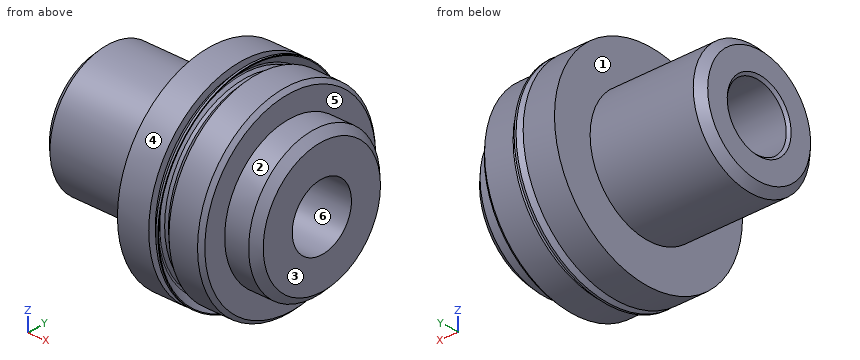
Autodesk Inventor part; units mm, degrees
ref_plane "hh_XY" through (0, 6.35, 0) normal (0, 0, 1) x (1, 0, 0)
ref_plane "hh_YZ" through (0, 6.35, 0) normal (1, 0, 0) x (0, 1, 0)
ref_plane "hh_ZX" through (0, 6.35, 0) normal (0, 1, 0) x (0, 0, 1)
sketch "Sketch_1" plane through (0, 0, 0) normal (0, 0, 1) x (1, 0, 0)
  line L0 (11.1252, 0) -> (0, 0)
  line L1 (0, 0) -> (0, 5.5944)
  line L2 (0, 5.5944) -> (0.7557, 6.35)
  line L3 (0.7557, 6.35) -> (11.1252, 6.35)
  line L4 (11.1252, 6.35) -> (11.1252, 0)
  line L5 (11.1252, 0) -> (0, 0)
revolve "Revolution1" add sketch "Sketch_1" angle 360 about axis through (11.1252, 0, 0) along (1, 0, 0)
thread "Thread1"
sketch "Sketch_3" plane through (0, 0, 0) normal (0, 0, 1) x (1, 0, 0)
  line L0 (19.05, 0) -> (11.1252, 0)
  line L1 (11.1252, 0) -> (11.1252, 10.2235)
  line L2 (11.1252, 10.2235) -> (14.2748, 10.2235)
  line L3 (14.2748, 10.2235) -> (14.2748, 8.9091)
  line L4 (14.2748, 8.9091) -> (15.0368, 8.9091)
  line L5 (15.0368, 8.9091) -> (15.7988, 9.671)
  line L6 (15.7988, 9.671) -> (18.669, 9.671)
  line L7 (18.669, 9.671) -> (19.05, 9.2901)
  line L8 (19.05, 9.2901) -> (19.05, 0)
  line L9 (19.05, 0) -> (11.1252, 0)
revolve "Revolution2" add sketch "Sketch_3" angle 360 about axis through (19.05, 0, 0) along (1, 0, 0)
sketch "Sketch_4" plane through (0, 0, 0) normal (0, 0, 1) x (1, 0, 0)
  line L0 (22.225, 0) -> (19.05, 0)
  line L1 (19.05, 0) -> (19.05, 7.1374)
  line L2 (19.05, 7.1374) -> (21.463, 7.1374)
  line L3 (21.463, 7.1374) -> (22.225, 6.3754)
  line L4 (22.225, 6.3754) -> (22.225, 0)
  line L5 (22.225, 0) -> (19.05, 0)
revolve "Revolution3" add sketch "Sketch_4" angle 360 about axis through (22.225, 0, 0) along (1, 0, 0)
sketch "Sketch4" plane through (0, 0, 0) normal (-1, 0, 0) x (0, 0, 1)
  point P0 (0, 0)
hole "Hole1" at (0, 0, 0) direction (1, 0, 0) diameter 6.4389 depth 22.225 countersink diameter 6.9469 countersink angle 90
sketch "Sketch_47" plane through (0, 0, 0) normal (0, 0, 1) x (1, 0, 0)
  line L0 (15.0368, 0) -> (14.2748, 0)
  line L1 (14.2748, 9.512) -> (14.2748, 8.655)
  line L2 (14.2748, 8.655) -> (15.0368, 8.655)
  line L3 (15.0368, 8.655) -> (15.0368, 8.9091)
  line L4 (15.0368, 8.9091) -> (14.6558, 8.9091)
  line L5 (14.6558, 8.9091) -> (14.3973, 9.1676)
  arc A0 (14.3973, 9.3472) -> (14.3973, 9.1676) centre (14.4871, 9.2574) ccw
  line L6 (14.3973, 9.3472) -> (15.1895, 10.1393)
  line L7 (15.1895, 10.1393) -> (15.1895, 10.2235)
  line L8 (15.1895, 10.2235) -> (14.9863, 10.2235)
  line L9 (14.9863, 10.2235) -> (14.2748, 9.512)
revolve "Revolution4" add sketch "Sketch_47" angle 360 about axis through (15.0368, 0, 0) along (1, 0, 0)
ref_plane "hh_XY" through (0, 6.35, 0) normal (0, 0, 1) x (1, 0, 0)
ref_plane "hh_YZ" through (0, 6.35, 0) normal (1, 0, 0) x (0, 1, 0)
ref_plane "hh_ZX" through (0, 6.35, 0) normal (0, 1, 0) x (0, 0, 1)
ref_plane "rod_guide_XY" through (0, 0, 0) normal (1, 0, 0) x (0, 0, -1)
ref_plane "rod_guide_YZ" through (0, 0, 0) normal (0, 0, -1) x (0, 1, 0)
ref_plane "rod_guide_ZX" through (0, 0, 0) normal (0, 1, 0) x (1, 0, 0)
ref_plane "t1_XY" through (11.1252, 0, 0) normal (1, 0, 0) x (0, 0, -1)
ref_plane "t1_YZ" through (11.1252, 0, 0) normal (0, 0, -1) x (0, 1, 0)
ref_plane "t1_ZX" through (11.1252, 0, 0) normal (0, 1, 0) x (1, 0, 0)
ref_plane "t111_XY" through (11.1252, 0, 0) normal (1, 0, 0) x (0, 0, -1)
ref_plane "t111_YZ" through (11.1252, 0, 0) normal (0, 0, -1) x (0, 1, 0)
ref_plane "t111_ZX" through (11.1252, 0, 0) normal (0, 1, 0) x (1, 0, 0)
ref_plane "to_foot_bracket_XY" through (11.1252, 0, 0) normal (1, 0, 0) x (0, 0, -1)
ref_plane "to_foot_bracket_YZ" through (11.1252, 0, 0) normal (0, 0, -1) x (0, 1, 0)
ref_plane "to_foot_bracket_ZX" through (11.1252, 0, 0) normal (0, 1, 0) x (1, 0, 0)
ref_plane "to_nut_XY" through (11.1252, 0, 0) normal (1, 0, 0) x (0, 0, -1)
ref_plane "to_nut_YZ" through (11.1252, 0, 0) normal (0, 0, -1) x (0, 1, 0)
ref_plane "to_nut_ZX" through (11.1252, 0, 0) normal (0, 1, 0) x (1, 0, 0)
ref_plane "to_rod_XY" through (0, 0, 0) normal (1, 0, 0) x (0, 0, -1)
ref_plane "to_rod_YZ" through (0, 0, 0) normal (0, 0, -1) x (0, 1, 0)
ref_plane "to_rod_ZX" through (0, 0, 0) normal (0, 1, 0) x (1, 0, 0)
ref_plane "to_screw_XY" through (6.35, 2.032, -6.0452) normal (0, 1, 0) x (1, 0, 0)
ref_plane "to_screw_YZ" through (6.35, 2.032, -6.0452) normal (1, 0, 0) x (0, 0, -1)
ref_plane "to_screw_ZX" through (6.35, 2.032, -6.0452) normal (0, 0, -1) x (0, 1, 0)
ref_plane "to_trunnion_brackets_XY" through (11.1252, 0, 0) normal (0, 1, 0) x (1, 0, 0)
ref_plane "to_trunnion_brackets_YZ" through (11.1252, 0, 0) normal (1, 0, 0) x (0, 0, -1)
ref_plane "to_trunnion_brackets_ZX" through (11.1252, 0, 0) normal (0, 0, -1) x (0, 1, 0)
ref_plane "to_trunnion_brackets1_XY" through (11.1252, 12.7, 0) normal (0, 1, 0) x (1, 0, 0)
ref_plane "to_trunnion_brackets1_YZ" through (11.1252, 12.7, 0) normal (1, 0, 0) x (0, 0, -1)
ref_plane "to_trunnion_brackets1_ZX" through (11.1252, 12.7, 0) normal (0, 0, -1) x (0, 1, 0)
ref_plane "to_trunnion_brackets2_XY" through (11.1252, -12.7, 0) normal (0, 1, 0) x (1, 0, 0)
ref_plane "to_trunnion_brackets2_YZ" through (11.1252, -12.7, 0) normal (1, 0, 0) x (0, 0, -1)
ref_plane "to_trunnion_brackets2_ZX" through (11.1252, -12.7, 0) normal (0, 0, -1) x (0, 1, 0)
ref_plane "to_tube_XY" through (15.0368, 0, 0) normal (1, 0, 0) x (0, 0, -1)
ref_plane "to_tube_YZ" through (15.0368, 0, 0) normal (0, 0, -1) x (0, 1, 0)
ref_plane "to_tube_ZX" through (15.0368, 0, 0) normal (0, 1, 0) x (1, 0, 0)
properties part number "04000-0_rod_guide"
Can you work these out from the model? Positions are in its coordinate system, mm. Face numbers are marked on the shaded views. A direction names the side the tool comes from. Give positions to 0.01 mm unless a question says otherwise; leave off trailing zeros. Order: outer loops, then holes, each group sorted by start corner. A loop starts at its lowest first (then second) coordinate and runs counter-clockwise, first axis right, second up. Notation, with made-up numbers: M -17.75,63.25 L 36.25,63.25 A27 ccw 36.25,89.25 Z; hole C -36.75,40 d11. An arc over 180 degrees is marked long. One line per item, written item: value.
Item 1: For the marked faces 1, 2 and 3, which set-ups out of +Z, -Z, +X, -X, +Y, -Y let a thin tool reach every point of the face, with its end or its side?
Verdict:
face 1: -X
face 2: +X
face 3: +Z, -Z, +X, +Y, -Y
Item 2: If we section it at A-A on x = 4.25: Write out the boundary of the cut face in (y, z).
Verdict:
outline: C 0,0 d12.7; hole C 0,0 d6.44
Item 3: If we mould it in two halves opening along Y, with no side actions, what happens to the marked faces 4, 5 and 6? For each: pulls with the +Y half, pulls with the -Y half, needs draft (parallel to the pull), parting line crosses it, or undercut.
Verdict:
face 4: parting line crosses it
face 5: needs draft
face 6: undercut
Item 4: Please list where these lines run through material, in increasing order: line 1 (Z direction, x = 11.75, y = 0); line 2 (Z direction, x = 16.5, y = 0); line 3 (Y direction, x = 15, z = 7.25).
Verdict:
line 1: -10.22 to -3.22, 3.22 to 10.22
line 2: -9.67 to -3.22, 3.22 to 9.67
line 3: -7.21 to -6.81, -5.18 to 5.18, 6.81 to 7.21
Item 5: For pin 1 (12 mm diameter, centred on x = 11, z = 8, fed in from +Y); pin 2 (8 mm diameter, centred on x = 3, y = 2, fed in from -Z); pin 3 (10 mm diameter, centred on x = 3, z = -2, fed in from +Y); pin 4 (5 mm diameter, centred on y = 0, z = 0, fed in from -X), each with a flat end and sliding along its axis, tell me the tip position at first contact or that it passes through.
Verdict:
pin 1: y = 10.03
pin 2: z = -6.35
pin 3: y = 6.35
pin 4: through
Item 6: If we section it at B-B on x = 11.75: Write out the boundary of the cut face in (y, z).
Verdict:
outline: C 0,0 d20.45; hole C 0,0 d6.44
